Work out the finished part from the listing and answer in its coordinate system (mm). A direction names the side the tool comes from. Give positions to 0.01 mm unless a question says otherwise; leave off trailing zeros. Order: outer loops, then holes, each group sorted by start corner. A loop starts at its lowest first (then second) coordinate and runs counter-clockwise, first axis right, second up.
```python
from build123d import *

# Parameters (mm, degrees)
EXTRUDE_1_DEPTH              = 2.9
SKETCH_2_R                   = 3.5
EXTRUDE_3_DEPTH              = 5
FILLET_1_R                   = 2
FILLET_2_R                   = 0.2
HOLE_WIZARD_M4_2_D           = 3.3
HOLE_WIZARD_M4_2_DEPTH       = 10.1
HOLE_WIZARD_M4_2_CSINK_D     = 4.05
HOLE_WIZARD_M4_2_CSINK_ANGLE = 90
HOLE_WIZARD_M4_2_TIP         = 0.991420021


with BuildPart() as part:
    # 草图1 → 凸台-拉伸1 (new body)
    with BuildSketch(Plane.XY):
        Polygon((3.067162176, -2.631700879), (3.812700905, 1.340389922), (0.745538729, 3.972090802), (-3.067162176, 2.631700879), (-3.812700905, -1.340389922), (-0.745538729, -3.972090802), align=None)
    extrude(amount=EXTRUDE_1_DEPTH)

    # 草图2 → 凸台-拉伸3 (add)
    with BuildSketch(Plane.XY.offset(2.9)):
        Circle(SKETCH_2_R)
    extrude(amount=-EXTRUDE_3_DEPTH)

    # 圆角1
    fillet_1_edges = [part.edges().sort_by_distance(p)[0] for p in [
        (-3.5, 0, -2.1),
    ]]
    fillet(fillet_1_edges, radius=FILLET_1_R)

    # 圆角2
    fillet_2_edges = [part.edges().sort_by_distance(p)[0] for p in [
        (-0.745538729, -3.972090802, 1.45),
        (-3.812700905, -1.340389922, 1.45),
        (-3.067162176, 2.631700879, 1.45),
        (0.745538729, 3.972090802, 1.45),
        (3.812700905, 1.340389922, 1.45),
        (3.067162176, -2.631700879, 1.45),
    ]]
    fillet(fillet_2_edges, radius=FILLET_2_R)

    # M4 螺纹孔2
    with Locations(Plane.XY.offset(2.9)):
        with Locations((0, 0)):
            CounterSinkHole(HOLE_WIZARD_M4_2_D / 2, HOLE_WIZARD_M4_2_CSINK_D / 2, depth=HOLE_WIZARD_M4_2_DEPTH, counter_sink_angle=HOLE_WIZARD_M4_2_CSINK_ANGLE)
            with Locations((0, 0, -(HOLE_WIZARD_M4_2_DEPTH + HOLE_WIZARD_M4_2_TIP / 2))):  # 118° drill point
                Cone(0, HOLE_WIZARD_M4_2_D / 2, HOLE_WIZARD_M4_2_TIP, mode=Mode.SUBTRACT)


solid = part.part
```
1. The part is cut by section A-A (z = 1.9). Write down the section's boundary in (x, y).
Findings below:
outline: (-3.79, -1.23) arc R0.2 ccw to (-3.73, -1.42) - (-0.83, -3.9) arc R0.2 ccw to (-0.64, -3.93) - (2.96, -2.67) arc R0.2 ccw to (3.09, -2.52) - (3.79, 1.23) arc R0.2 ccw to (3.73, 1.42) - (0.83, 3.9) arc R0.2 ccw to (0.64, 3.93) - (-2.96, 2.67) arc R0.2 ccw to (-3.09, 2.52) - close; hole circle Ø3.3 at (0, 0)
2. Which of the six approach directions +Z, -Z, +X, -X, +Y, -Y give full straight-line access (tool end or side, diameter ignored) to faces 4 (the face through (2.8, -2.4, 0)), 5 (the face through (-1.14, 3.31, 1.43))?
Findings below:
face 4: -Z, +X, -Y
face 5: +Z, -Z, -X, +Y
3. Straight lines are drawn through the part: probe 1 along Y at (x, z) = (0, -0.15); probe 2 along X at (y, z) = (1, 2.5); probe 3 along Y at (x, z) = (0, 0.95). For each, find the intervals that lie inside material, in ascending order.
Findings below:
probe 1: y = -3.5 to -1.65, 1.65 to 3.5
probe 2: x = -3.37 to -1.31, 1.31 to 3.75
probe 3: y = -3.71 to -1.65, 1.65 to 3.71
4. The mould has two halves that part along X. Classify faces 1 (the face through (-2.8, 2.4, 0)), 2 (the face through (1.14, -3.31, 1.43)), 3 (the face through (1.216, 1.115, 0.183)): pulls with the +X half, pulls with the -X half, needs draft (parallel to the pull), parting line crosses it, or undercut.
Findings below:
face 1: needs draft
face 2: pulls with the +X half
face 3: undercut
5. Given P1, Ø0.7, axis at x = 2.5, y = -1.5, coming from the -Z side; P2, Ø0.5, axis at x = 3, y = 1, coming from the -Z side; P3, Ø4, axis at x = 0, y = 0, coming from the +Z side (3 decimals), each flat-ended and moving along its own axis, determine where each tip first touches the part or whether it passes through.
Findings below:
P1: stops at z = -1.79
P2: stops at z = -1.52
P3: stops at z = 2.875
